Autodesk Inventor part; units mm, degrees
ref_plane "to_blackets_XY" through (3.9, 0, 2.5) normal (1, 0, 0) x (0, 0, -1)
ref_plane "to_blackets_YZ" through (3.9, 0, 2.5) normal (0, 0, -1) x (0, 1, 0)
ref_plane "to_blackets_ZX" through (3.9, 0, 2.5) normal (0, 1, 0) x (1, 0, 0)
sketch "_____2" plane through (0, 0, 0) normal (0, 0, 1) x (1, 0, 0)
  arc A0 (0, -1.7352) -> (0.1786, -2.1182) centre (0.5, -1.7352) ccw
  line L0 (0.1786, -2.1182) -> (2.4606, -4.033)
  arc A1 (2.4606, -4.033) -> (2.782, -4.15) centre (2.782, -3.65) ccw
  line L1 (2.782, -4.15) -> (3, -4.15)
  arc A2 (3, -4.15) -> (3.2, -3.95) centre (3, -3.95) ccw
  line L2 (3.2, -3.95) -> (3.2, -3.1)
  arc A3 (3.4, -2.9) -> (3.2, -3.1) centre (3.4, -3.1) ccw
  line L3 (3.4, -2.9) -> (3.7, -2.9)
  arc A4 (3.7, -2.9) -> (3.9, -2.7) centre (3.7, -2.7) ccw
  line L4 (3.9, -2.7) -> (3.9, 2.7)
  arc A5 (3.9, 2.7) -> (3.7, 2.9) centre (3.7, 2.7) ccw
  line L5 (3.7, 2.9) -> (3.4, 2.9)
  arc A6 (3.2, 3.1) -> (3.4, 2.9) centre (3.4, 3.1) ccw
  line L6 (3.2, 3.1) -> (3.2, 3.95)
  arc A7 (3.2, 3.95) -> (3, 4.15) centre (3, 3.95) ccw
  line L7 (3, 4.15) -> (2.782, 4.15)
  arc A8 (2.782, 4.15) -> (2.4606, 4.033) centre (2.782, 3.65) ccw
  line L8 (2.4606, 4.033) -> (0.1786, 2.1182)
  arc A9 (0.1786, 2.1182) -> (0, 1.7352) centre (0.5, 1.7352) ccw
  line L9 (0, 1.7352) -> (0, -1.7352)
extrude "Extrusion1" add sketch "_____2" along normal mid plane 17
sketch "Sketch_2" plane through (0, 0, 2.5) normal (0, 0, 1) x (1, 0, 0)
  line L0 (3.9, 0) -> (0, 0)
  line L1 (0, 0) -> (0, 2.5)
  line L2 (0, 2.5) -> (0.433, 2.067)
  line L3 (0.433, 2.067) -> (3.467, 2.067)
  line L4 (3.467, 2.067) -> (3.9, 2.5)
  line L5 (3.9, 2.5) -> (3.9, 0)
  line L6 (3.9, 0) -> (0, 0)
revolve "Revolution1" cut sketch "Sketch_2" angle 360 about axis through (3.9, 0, 2.5) along (1, 0, 0)
thread "Thread1"
sketch "_____1" plane through (0, 0, -4.5) normal (0, 0, 1) x (1, 0, 0)
  line L0 (0.95, 0) -> (0, 0)
  line L1 (0, 0) -> (0, 1.75)
  line L2 (0, 1.75) -> (0.95, 1.75)
  line L3 (0.95, 1.75) -> (0.95, 0)
  line L4 (0.95, 0) -> (0, 0)
revolve "Revolution2" cut sketch "_____1" angle 360 about axis through (0.95, 0, -4.5) along (1, 0, 0)
sketch "Sketch_3" plane through (0, 0, -4.5) normal (0, 0, 1) x (1, 0, 0)
  line L0 (2.7, 0) -> (-0.8, 0)
  arc A0 (2.7, 0) -> (-0.8, 0) centre (0.95, 0) ccw
  line L1 (2.7, 0) -> (-0.8, 0)
revolve "Revolution3" add sketch "Sketch_3" angle 360 about axis through (2.7, 0, -4.5) along (1, 0, 0)
ref_plane "to_blackets_XY" through (3.9, 0, 2.5) normal (1, 0, 0) x (0, 0, -1)
ref_plane "to_blackets_YZ" through (3.9, 0, 2.5) normal (0, 0, -1) x (0, 1, 0)
ref_plane "to_blackets_ZX" through (3.9, 0, 2.5) normal (0, 1, 0) x (1, 0, 0)
ref_plane "to_bolt_XY" through (0, 0, 2.5) normal (1, 0, 0) x (0, 0, -1)
ref_plane "to_bolt_YZ" through (0, 0, 2.5) normal (0, 0, -1) x (0, 1, 0)
ref_plane "to_bolt_ZX" through (0, 0, 2.5) normal (0, 1, 0) x (1, 0, 0)
ref_plane "to_frames_XY" through (3.2, 0, 2.5) normal (1, 0, 0) x (0, 0, -1)
ref_plane "to_frames_YZ" through (3.2, 0, 2.5) normal (0, 0, -1) x (0, 1, 0)
ref_plane "to_frames_ZX" through (3.2, 0, 2.5) normal (0, 1, 0) x (1, 0, 0)
properties part number "HNTP5-5"
Here's how the part is built. I have some questions about the finished solid (model axes, mm). A direction names the side the tool comes from. Coordinates: 2 decimals unless noted, no trailing zeros. Loops run counter-clockwise (first coordinate to the right, second up) from the corner with the lowest first, then second, coordinate; pieces in that order, holes last.
1. Imagine slicing it at C-C, the plane z = 2.5. Please give me the cut outline in (x, y).
2. For P1, Ø1, axis at y = 0, z = -2, coming from the -X side; P2, Ø0.9, axis at y = 3.5, z = 1, coming from the +X side; P3, Ø3, axis at y = 0, z = -7, coming from the -X side, each with a flat end and sliding along its axis, tell me the tip position at first contact or that it passes through.
3. Imagine slicing it at D-D, the plane x = 2.05. Please give me the cut outline in (y, z), and give its area (3 significant figures).
4. Imagine slicing it at A-A, the plane y = 0. Please give me the cut outline in (x, z), and give its area (3 significant figures).
5. If we mould it in two halves opening along Z, with no side actions, what happens to faces 1 (the flat face through (2, 0, 8.5)), 2 (the cylindrical face through (1.971, -0.448, 0.482)), 3 (the flat face through (3.9, -1, 0)), 4 (the flat face through (2, 0, -8.5))? For each: pulls with the +Z half, pulls with the -Z half, needs draft (parallel to the pull), parting line crosses it, or undercut.
6. Imagine slicing it at B-B, the plane z = 6. Please give me the cut outline in (x, y).
7. For faces 5 (the flat face through (0, 0, 6)), 6 (the flat face through (3.2, -3.5, -0.1)), 7 (the flat face through (3.2, 3.5, -0.1)), 8 (the flat face through (1.336, 3.089, -0.119)), which set-ups out of +Z, -Z, +X, -X, +Y, -Y let a thin tool reach every point of the face, with its end or its side?
8. I need wall thicknesses on L1, parallel to X at y = 1, z = -2; L2, parallel to Y at x = 3.65, z = -7.5; L3, parallel to Z at x = 3.3, y = 0.5. Which ranges of each line are inside material? Lowest first, please.
Taken from the geometry:
1. outline: (0.29, -2.21) - (2.46, -4.03) arc R0.5 ccw to (2.78, -4.15) - (3, -4.15) arc R0.2 ccw to (3.2, -3.95) - (3.2, -3.1) arc R0.2 cw to (3.4, -2.9) - (3.7, -2.9) arc R0.2 ccw to (3.9, -2.7) - (3.9, -2.5) - (3.47, -2.07) - (0.43, -2.07) - close; (0.29, 2.21) - (0.43, 2.07) - (3.47, 2.07) - (3.9, 2.5) - (3.9, 2.7) arc R0.2 ccw to (3.7, 2.9) - (3.4, 2.9) arc R0.2 cw to (3.2, 3.1) - (3.2, 3.95) arc R0.2 ccw to (3, 4.15) - (2.78, 4.15) arc R0.5 ccw to (2.46, 4.03) - close
2. P1: stops at x = 0
2. P2: stops at x = 3.21
2. P3: stops at x = -0.49
3. outline: (-3.69, -8.5) - (3.69, -8.5) - (3.69, 8.5) - (-3.69, 8.5) - close; hole circle Ø4.13 at (0, 2.5)
3. area: 112 mm2
4. outline: (0, -8.5) - (3.9, -8.5) - (3.9, 0) - (3.47, 0.43) - (0.43, 0.43) - (0, 0) - (0, -2.75) - (0.95, -2.75) arc R1.75 ccw to (0.95, -6.25) - (0, -6.25) - close; (0, 5) - (0.43, 4.57) - (3.47, 4.57) - (3.9, 5) - (3.9, 8.5) - (0, 8.5) - close
4. area: 51.3 mm2
5. face 1: pulls with the +Z half
5. face 2: undercut
5. face 3: needs draft
5. face 4: pulls with the -Z half
6. outline: (0, -1.74) arc R0.5 ccw to (0.18, -2.12) - (2.46, -4.03) arc R0.5 ccw to (2.78, -4.15) - (3, -4.15) arc R0.2 ccw to (3.2, -3.95) - (3.2, -3.1) arc R0.2 cw to (3.4, -2.9) - (3.7, -2.9) arc R0.2 ccw to (3.9, -2.7) - (3.9, 2.7) arc R0.2 ccw to (3.7, 2.9) - (3.4, 2.9) arc R0.2 cw to (3.2, 3.1) - (3.2, 3.95) arc R0.2 ccw to (3, 4.15) - (2.78, 4.15) arc R0.5 ccw to (2.46, 4.03) - (0.18, 2.12) arc R0.5 ccw to (0, 1.74) - close
7. face 5: +Z, -X, +Y, -Y
7. face 6: +Z, -Z, +X, -Y
7. face 7: +Z, -Z, +X, +Y
7. face 8: +Z, -Z, -X, +Y
8. L1: x = 0 to 3.9
8. L2: y = -2.9 to 2.9
8. L3: z = -8.5 to 0.49, 4.51 to 8.5
